Source: CAD feature listing. Evaluate the final solid. Frame: model axes, mm. A direction names the side the tool comes from. Coordinates: 2 decimals unless noted, no trailing zeros. Order: outer loops, then holes, each group sorted by start corner. A loop starts at its lowest first (then second) coordinate and runs counter-clockwise, first axis right, second up. Notation, with made-up numbers: (-21, 67) -> (-1, 67) arc R27 ccw to (-1, 83) -> close; hole circle Ø7 at (19, 78.5). An arc over 180 degrees is marked (long way). Put each result on its own line as item: value.
Autodesk Inventor part; units mm, degrees
ref_plane "Work Plane1" through (-4.1, 42.6608, -9.2) normal (0, 1, 0) x (0, 0, 1)
ref_plane "YZ Plane" through (0, 0, 0) normal (1, 0, 0) x (0, 1, 0)
ref_plane "XZ Plane" through (0, 0, 0) normal (0, 1, 0) x (-1, 0, 0)
sketch "Sketch1" plane through (0, 0, 0) normal (0, 0, 1) x (1, 0, 0)
  line L0 (22.8, 0) -> (0, 0)
  line L1 (22.8, 12.5) -> (22.8, 0)
  line L2 (0, 12.5) -> (22.8, 12.5)
  line L3 (0, 0) -> (0, 12.5)
  arc A0 (-3.7, 5.65) -> (-3.7, 6.85) centre (-2.9, 6.25) ccw
  arc A1 (26.5, 6.85) -> (26.5, 5.65) centre (25.7, 6.25) ccw
  line L4 (23.2, 12.9) -> (23.2, -0.4)
  line L5 (23.2, -0.4) -> (-0.4, -0.4)
  line L6 (-0.4, -0.4) -> (-0.4, 12.9)
  line L7 (-0.4, 12.9) -> (23.2, 12.9)
  line L8 (27.6, 6.85) -> (27.6, 12.5) construction
  line L9 (27.629, -4.829) -> (27.629, 17.329)
  line L10 (27.629, 17.329) -> (-4.829, 17.329)
  line L11 (-4.829, 17.329) -> (-4.829, -4.829)
  line L12 (-4.829, -4.829) -> (27.629, -4.829)
  arc A2 (-4.1, 5.35) -> (-4.1, 7.15) centre (-2.9, 6.25) ccw
  arc A3 (26.9, 7.15) -> (26.9, 5.35) centre (25.7, 6.25) ccw
  circle A4 centre (-2.9, 6.25) radius 1.5
  circle A5 centre (25.7, 6.25) radius 1.5
  dimension "d0" = 0.4
  dimension "d1" = 0.5
  dimension "d2" = 0.5
extrude "Extrusion1" add sketch "Sketch1" along normal blind 3 contours L12 L11 L10 L9
sketch "Sketch2" plane through (-4.829, -4.829, 0) normal (0, -1, 0) x (1, 0, 0)
  line L0 (0, 0) -> (32.458, 0)
  line L1 (32.458, 0) -> (32.458, 3)
  line L2 (0, 3) -> (32.458, 3)
  line L3 (0, 0) -> (0, 3)
  point P0 (4.829, 0)
extrude "Extrusion2" cut sketch "Sketch2" against normal blind 4.6
sketch "Sketch3" plane through (-4.829, 17.329, 0) normal (0, 1, 0) x (1, 0, 0)
  line L0 (32.458, -3) -> (0, -3)
  line L1 (0, 0) -> (7, 0)
  line L2 (7, 0) -> (7, -3)
  line L3 (7, -3) -> (0, -3)
  line L4 (0, -3) -> (0, 0)
  point P0 (4.829, 0)
  dimension "d7" = 7
ref_plane "Work Plane1" through (-4.1, 42.6608, -9.2) normal (0, 1, 0) x (0, 0, 1)
extrude "Extrusion3" add sketch "Sketch3" along normal up to surface (25.3318 mm away)
sketch "Sketch4" plane through (0, 0, 0) normal (0, 0, -1) x (-1, 0, 0)
  circle A0 centre (2.1, 37.6608) radius 2
  line L0 (-1.9, 39.6608) -> (-1.9, 32.6608)
  line L1 (-6.3422, 39.6608) -> (-1.9, 39.6608)
  line L2 (-6.3422, 39.6608) -> (-6.3422, 42.6608)
  line L3 (-6.3422, 42.6608) -> (4.1, 42.6608)
  arc A1 (6.1, 40.6608) -> (4.1, 42.6608) centre (4.1, 40.6608) ccw
  line L4 (6.1, 32.6608) -> (6.1, 40.6608)
  line L5 (-1.9, 32.6608) -> (6.1, 32.6608)
  point P0 (0, 0)
extrude "Extrusion4" add sketch "Sketch4" along normal up to surface (4.2 mm away)
sketch "Sketch5" plane through (0, 0, 0) normal (0, 0, 1) x (1, 0, 0)
  line L0 (2.171, 39.6608) -> (2.171, 42.6608)
  line L1 (6.3422, 39.6608) -> (2.171, 39.6608)
  line L2 (6.3422, 42.6608) -> (6.3422, 39.6608)
  line L3 (2.171, 42.6608) -> (6.3422, 42.6608)
  point P0 (0, 0)
extrude "Extrusion5" cut sketch "Sketch5" against normal up to surface (4.2 mm away)
sketch "Sketch6" plane through (0, 0, 0) normal (0, 0, 1) x (1, 0, 0)
  line L0 (-4.829, 32.6608) -> (-4.829, 42.5232)
  arc A0 (-4.829, 42.5232) -> (-6.1, 40.6608) centre (-4.1, 40.6608) ccw
  line L1 (-6.1, 32.6608) -> (-6.1, 40.6608)
  line L2 (-4.829, 32.6608) -> (-6.1, 32.6608)
  point P0 (0, 0)
extrude "Extrusion6" add sketch "Sketch6" along normal up to surface (3 mm away)
sketch "Sketch7" plane through (1.9, 32.6608, 0) normal (1, 0, 0) x (0, 0, -1)
  line L0 (4.2, 0) -> (4.2, 7)
  line L1 (0, 7) -> (4.2, 7)
  line L2 (0, 0) -> (0, 7)
  line L3 (0, 0) -> (4.2, 0)
  point P0 (0, -32.6608)
extrude "Extrusion7" add sketch "Sketch7" along normal up to surface (0.271 mm away)
sketch "Sketch8" plane through (-6.1, 32.6608, -4.2) normal (-1, 0, 0) x (0, 0, 1)
  line L0 (2, 8.75) -> (5.5, 8.75)
  line L1 (5.5, 8.75) -> (5.5, 1.25)
  line L2 (5.5, 1.25) -> (2, 1.25)
  line L3 (2, 1.25) -> (2, 8.75)
  line L4 (0, 7) -> (0, 3) construction
  line L5 (0, 7) -> (0, 3) construction
  line L6 (4.2, 7) -> (4.2, 3) construction
  line L7 (4.2, 7) -> (0, 7) construction
  line L8 (4.2, 3) -> (0, 3) construction
  point P0 (4.2, -32.6608)
  dimension "d19" = 3.5
  dimension "d20" = 7.5
  dimension "d21" = 1.75
  dimension "d22" = 2
extrude "Extrusion8" cut sketch "Sketch8" against normal through all
sketch "Sketch9" plane through (-6.1, 33.9108, 1.3) normal (0, 0, -1) x (-1, 0, 0)
  circle A0 centre (-4, 3.75) radius 2
  circle A1 centre (-4, 3.75) radius 2.2
  point P0 (-6.1, -33.9108)
  dimension "d25" = 0.2
extrude "Extrusion9" cut sketch "Sketch9" along normal through all both and the other way through all contours A0 | A1
sketch "Sketch10" plane through (-4.829, 32.6608, 0) normal (0, -1, 0) x (1, 0, 0)
  line L0 (-1.271, -4.2) -> (7, -4.2)
  line L1 (7, -4.2) -> (7, 0)
  line L2 (0, 0) -> (7, 0)
  line L3 (0, 3) -> (0, 0)
  line L4 (0, 3) -> (-1.271, 3)
  line L5 (-1.271, 3) -> (-1.271, -4.2)
  point P0 (4.829, 0)
extrude "Extrusion10" add sketch "Sketch10" along normal blind 2
fillet "Fillet2" radius 1 2 edges at (-1.329, 30.6608, 0) (-4.829, 30.6608, 1.5)
properties part number "ServoBracket"
1. First-contact query: pin 1 (2 mm diameter, centred on y = 22, z = 0.5, fed in from +X); pin 2 (0.9 mm diameter, centred on y = 7.5, z = 1, fed in from -X); pin 3 (3.5 mm diameter, centred on x = -2.9, y = 6.25, fed in from +Z); pin 4 (1 mm diameter, centred on x = 24, y = 18, fed in from -Z). Flat tips, straight axial feed; report the tip coordinate or a pass-through.
Numbers:
pin 1: stops at x = 2.17
pin 2: stops at x = -4.83
pin 3: stops at z = 3
pin 4: passes through
2. Set-up query: faces 4 (the flat face through (15, 17.329, 1)), 5 (the flat face through (-4.829, 15, 2)), 6 (the flat face through (-2, 41.411, 0)), 7 (the flat face through (11, 12.9, 1)). Return all of +Z, -Z, +X, -X, +Y, -Y with unobstructed straight access to the full face (end or side cutting, diameter ignored); none if empty.
Numbers:
face 4: +Z, -Z, +X, +Y
face 5: +Z, -Z, -X, -Y
face 6: +X, -X
face 7: +Z, -Z, -Y
3. Cut plane A-A on y = 6.25. Output: boundary loops of the cut face in (x, z).
Numbers:
outline: (-4.83, 0) -> (-4.4, 0) -> (-4.4, 3) -> (-4.83, 3) -> close; (-1.4, 0) -> (-0.4, 0) -> (-0.4, 3) -> (-1.4, 3) -> close; (23.2, 0) -> (24.2, 0) -> (24.2, 3) -> (23.2, 3) -> close; (27.2, 0) -> (27.63, 0) -> (27.63, 3) -> (27.2, 3) -> close
4. Cut plane C-C on x = -2.1. Output: boundary loops of the cut face in (y, z).
Numbers:
outline: (-0.23, 0) -> (4.98, 0) -> (4.98, 3) -> (-0.23, 3) -> close; (7.52, 0) -> (29.66, 0) arc R1 cw to (30.66, -1) -> (30.66, -4.2) -> (35.46, -4.2) -> (35.46, -2.2) -> (33.91, -2.2) -> (33.91, 1.3) -> (35.46, 1.3) -> (35.46, 3) -> (7.52, 3) -> close; (39.86, -4.2) -> (42.66, -4.2) -> (42.66, 3) -> (39.86, 3) -> (39.86, 1.3) -> (41.41, 1.3) -> (41.41, -2.2) -> (39.86, -2.2) -> close
5. Ray query, line 1 along X through (y, z) = (6.25, 1.7); line 2 along Y through (x, z) = (1.5, 0.25); line 3 along Y through (x, z) = (-2.1, -3.8). Return the intervals inside material, ascending.
Numbers:
line 1: x = -4.83 to -4.4, -1.4 to -0.4, 23.2 to 24.2, 27.2 to 27.63
line 2: y = 12.9 to 33.91, 41.41 to 42.66
line 3: y = 30.66 to 35.46, 39.86 to 42.66
6. Cut plane D-D on z = -3. Output: boundary loops of the cut face in (x, y), plus the area to 3 significant figures.
Numbers:
outline: (-6.1, 30.66) -> (2.17, 30.66) -> (2.17, 42.66) -> (-4.1, 42.66) arc R2 ccw to (-6.1, 40.66) -> close; hole circle Ø4.4 at (-2.1, 37.66)
area: 83.2 mm2
7. Pull-direction query (Y, two-part tool) for faces 1 (the flat face through (25, -0.229, 2)), 2 (the flat face through (-4, 36, 1.3)), 3 (the flat face through (-2, 35, -4.2)); classes: pulls with the +Y half, pulls with the -Y half, needs draft (parallel to the pull), parting line crosses it, or undercut.
Numbers:
face 1: pulls with the -Y half
face 2: undercut
face 3: needs draft
8. Cut plane B-B on x = 25.7. Output: boundary loops of the cut face in (y, z).
Numbers:
outline: (-0.23, 0) -> (4.75, 0) -> (4.75, 3) -> (-0.23, 3) -> close; (7.75, 0) -> (17.33, 0) -> (17.33, 3) -> (7.75, 3) -> close
